```python
from build123d import *

# Parameters (mm, degrees)
CROQUIS1_W              = 52
CROQUIS1_H              = 37
SALIENTE_EXTRUIR1_DEPTH = 3
REDONDEO1_R             = 3
CROQUIS2_R              = 1.5
CORTAR_EXTRUIR1_DEPTH   = 3
CROQUIS3_W              = 29
CROQUIS3_H              = 20
CROQUIS3_W_2            = 6
CROQUIS3_H_2            = 14
CORTAR_EXTRUIR2_DEPTH   = 3
SALIENTE_EXTRUIR2_DEPTH = 9
CROQUIS5_W              = 36
CROQUIS5_H              = 28.002550662
SALIENTE_EXTRUIR3_DEPTH = 10.3
CORTAR_EXTRUIR3_START   = -28.002551
CORTAR_EXTRUIR3_DEPTH   = 28.002551
SALIENTE_EXTRUIR4_DEPTH = 8.5
CROQUIS8_W              = 21.9
CROQUIS8_H              = 60.9
CORTAR_EXTRUIR4_DEPTH   = 5.5
CORTAR_EXTRUIR5_DEPTH   = 9
CORTAR_EXTRUIR6_START   = -28.002551
CROQUIS12_W             = 9
CROQUIS12_H             = 1.570892211
CORTAR_EXTRUIR6_DEPTH   = 28.002551
CROQUIS13_W             = 3
CROQUIS13_H             = 67
SALIENTE_EXTRUIR5_DEPTH = 12
CORTAR_EXTRUIR7_START   = -28.002551
CROQUIS14_W             = 31
CROQUIS14_H             = 9
CORTAR_EXTRUIR7_DEPTH   = 28.002551
CROQUIS17_R             = 1.5
SALIENTE_EXTRUIR6_DEPTH = 9
CORTAR_EXTRUIR8_START   = -37
CROQUIS18_W             = 54.197150846
CROQUIS18_H             = 9
CORTAR_EXTRUIR8_DEPTH   = 37
CORTAR_EXTRUIR9_REACH   = 83.194
CROQUIS19_R             = 1.5
CROQUIS20_W             = 28
CROQUIS20_H             = 6
SALIENTE_EXTRUIR7_DEPTH = 3
CROQUIS21_W             = 20
CROQUIS21_H             = 4.5
CORTAR_EXTRUIR10_DEPTH  = 2
CROQUIS22_R             = 3
CORTAR_EXTRUIR11_DEPTH  = 10.3
CORTAR_EXTRUIR12_REACH  = 82.263
CROQUIS23_R             = 2


with BuildPart() as part:
    # Croquis1 → Saliente-Extruir1 (new body)
    with BuildSketch(Plane.XY):
        with Locations((-39.296803653, 6.787671233)):
            Rectangle(CROQUIS1_W, CROQUIS1_H)
    extrude(amount=SALIENTE_EXTRUIR1_DEPTH)

    # Redondeo1
    redondeo1_edges = [part.edges().sort_by_distance(p)[0] for p in [
        (-65.296803653, 25.287671233, 1.5),
        (-65.296803653, -11.712328767, 1.5),
    ]]
    fillet(redondeo1_edges, radius=REDONDEO1_R)

    # Croquis2 → Cortar-Extruir1 (cut)
    with BuildSketch(Plane.XY.offset(3)):
        with Locations((-61.296803653, 21.287671233)):
            Circle(CROQUIS2_R)
        with Locations((-61.296803653, -7.712328767)):
            Circle(CROQUIS2_R)
        with Locations((-16.624072342, -7.712328767)):
            Circle(CROQUIS2_R)
        with Locations((-17.296803653, 21.287671233)):
            Circle(CROQUIS2_R)
    extrude(amount=-CORTAR_EXTRUIR1_DEPTH, mode=Mode.SUBTRACT)

    # Croquis3 → Cortar-Extruir2 (cut)
    with BuildSketch(Plane.XY.offset(3)):
        with Locations((-50.796803653, 6.787671233)):
            Rectangle(CROQUIS3_W, CROQUIS3_H)
        with Locations((-16.296803653, 6.787671233)):
            Rectangle(CROQUIS3_W_2, CROQUIS3_H_2)
    extrude(amount=-CORTAR_EXTRUIR2_DEPTH, mode=Mode.SUBTRACT)

    # Croquis4 → Saliente-Extruir2 (add)
    with BuildSketch(Plane.XY.offset(3)):
        Polygon((-57.296803653, 16.787671233), (-57.296803653, 20.790221895), (-26.296803653, 20.790221895), (-26.296803653, -7.212328767), (-57.296803653, -7.212328767), (-57.296803653, -3.212328767), (-36.296803653, -3.212328767), (-36.296803653, 16.787671233), align=None)
    extrude(amount=SALIENTE_EXTRUIR2_DEPTH)

    # Croquis5 → Saliente-Extruir3 (add)
    with BuildSketch(Plane.XY.offset(12)):
        with Locations((-44.296803653, 6.788946564)):
            Rectangle(CROQUIS5_W, CROQUIS5_H)
    extrude(amount=SALIENTE_EXTRUIR3_DEPTH)

    # Croquis6 → Cortar-Extruir3 (cut)
    with BuildSketch(Plane.XZ.offset(7.212328767).offset(CORTAR_EXTRUIR3_START)):
        Polygon((-35.296803653, 15), (-35.296803653, 12.995381041), (-26.296803653, 12.995381041), (-26.296803653, 14.757444162), (-26.296803653, 22.3), (-62.296803653, 22.3), align=None)
    extrude(amount=CORTAR_EXTRUIR3_DEPTH, mode=Mode.SUBTRACT)

    # Croquis7 → Saliente-Extruir4 (add)
    with BuildSketch(Plane(origin=(1.374852463, 0, 5.085070754), x_dir=(0.9653390502996949, 0, -0.2609990765625102), z_dir=(0.2609990765625102, 0, 0.9653390502996949))):
        Polygon((-65.957816682, 6.788946564), (-65.957816682, -26.711053436), (-37.957816682, -26.711053436), (-37.957816682, 40.288946564), (-65.957816682, 40.288946564), align=None)
    extrude(amount=SALIENTE_EXTRUIR4_DEPTH)

    # Croquis8 → Cortar-Extruir4 (cut)
    with BuildSketch(Plane(origin=(3.593344614, 0, 13.290452681), x_dir=(0.9653390502996949, 0, -0.26099907656251026), z_dir=(0.26099907656251026, 0, 0.9653390502996949))):
        with Locations((-51.957816682, 6.788946564)):
            Rectangle(CROQUIS8_W, CROQUIS8_H)
    extrude(amount=-CORTAR_EXTRUIR4_DEPTH, mode=Mode.SUBTRACT)

    # Croquis10 → Cortar-Extruir5 (cut)
    with BuildSketch(Plane(origin=(0, 20.790221895, 0), x_dir=(1, 0, 0), z_dir=(0, 1, 0))):
        Polygon((-62.296803653, -22.3), (-35.296803653, -15), (-35.296803653, -12), (-62.296803653, -19.3), align=None)
    extrude(amount=-CORTAR_EXTRUIR5_DEPTH, mode=Mode.SUBTRACT)

    # Croquis12 → Cortar-Extruir6 (cut)
    with BuildSketch(Plane(origin=(0, 20.790221895, 0), x_dir=(1, 0, 0), z_dir=(0, 1, 0)).offset(CORTAR_EXTRUIR6_START)):
        with Locations((-30.796803653, -12.209934936)):
            Rectangle(CROQUIS12_W, CROQUIS12_H)
    extrude(amount=CORTAR_EXTRUIR6_DEPTH, mode=Mode.SUBTRACT)

    # Croquis13 → Saliente-Extruir5 (add)
    with BuildSketch(Plane(origin=(3.593344614, 0, 13.290452681), x_dir=(0.9653390502996949, 0, -0.26099907656251026), z_dir=(0.26099907656251026, 0, 0.9653390502996949))):
        with Locations((-39.457816682, 6.788946564)):
            Rectangle(CROQUIS13_W, CROQUIS13_H)
    extrude(amount=SALIENTE_EXTRUIR5_DEPTH)

    # Croquis14 → Cortar-Extruir7 (cut)
    with BuildSketch(Plane.XZ.offset(7.212328767).offset(CORTAR_EXTRUIR7_START)):
        with Locations((-41.796803653, 7.5)):
            Rectangle(CROQUIS14_W, CROQUIS14_H)
    extrude(amount=CORTAR_EXTRUIR7_DEPTH, mode=Mode.SUBTRACT)


with BuildPart() as cortar_extruir7_piece_1:
    # of the separate pieces the step leaves, piece 1, a body of its own (cortar_extruir7_pieces)
    add(part.part.solids().sort_by_distance((-62.296803653, -26.711053436, 22.3))[0])



with BuildPart() as cortar_extruir7_piece_2:
    # of the separate pieces the step leaves, piece 2, a body of its own (cortar_extruir7_pieces)
    add(part.part.solids().sort_by_distance((-62.296803653, 25.287671233, 3))[0])


with BuildPart() as cortar_extruir7_piece_1_1:
    add(cortar_extruir7_piece_1.part)

    add(cortar_extruir7_piece_2.part)  # Saliente-Extruir6 merges Cortar-Extruir7 piece 2
    # Croquis17 → Saliente-Extruir6 (add)
    with BuildSketch(Plane.XY.offset(3)):
        with BuildLine():
            Line((-13.296803653, -0.212328767), (-19.296803653, -0.212328767))
            Line((-19.296803653, -0.212328767), (-19.296803653, 13.787671233))
            Line((-19.296803653, 13.787671233), (-13.296803653, 13.787671233))
            Line((-13.296803653, 13.787671233), (-13.296803653, 25.287671233))
            Line((-13.296803653, 25.287671233), (-62.296803653, 25.287671233))
            ThreePointArc((-62.296803653, 25.287671233), (-64.418123997, 24.408991576), (-65.296803653, 22.287671233))
            Line((-65.296803653, 22.287671233), (-65.296803653, 16.787671233))
            Line((-65.296803653, 16.787671233), (-36.296803653, 16.787671233))
            Line((-36.296803653, 16.787671233), (-36.296803653, -3.212328767))
            Line((-36.296803653, -3.212328767), (-65.296803653, -3.212328767))
            Line((-65.296803653, -3.212328767), (-65.296803653, -8.712328767))
            ThreePointArc((-65.296803653, -8.712328767), (-64.418123997, -10.833649111), (-62.296803653, -11.712328767))
            Line((-62.296803653, -11.712328767), (-13.296803653, -11.712328767))
            Line((-13.296803653, -11.712328767), (-13.296803653, -0.212328767))
        make_face()
        with Locations((-61.296803653, 21.287671233)):
            Circle(CROQUIS17_R, mode=Mode.SUBTRACT)
        with Locations((-61.296803653, -7.712328767)):
            Circle(CROQUIS17_R, mode=Mode.SUBTRACT)
        with Locations((-16.624072342, -7.712328767)):
            Circle(CROQUIS17_R, mode=Mode.SUBTRACT)
        with Locations((-17.296803653, 21.287671233)):
            Circle(CROQUIS17_R, mode=Mode.SUBTRACT)
    extrude(amount=SALIENTE_EXTRUIR6_DEPTH)

    # Croquis18 → Cortar-Extruir8 (cut)
    with BuildSketch(Plane.XZ.offset(11.712328767).offset(CORTAR_EXTRUIR8_START)):
        with Locations((-40.395379076, 4.5)):
            Rectangle(CROQUIS18_W, CROQUIS18_H)
    extrude(amount=CORTAR_EXTRUIR8_DEPTH, mode=Mode.SUBTRACT)

    # Cortar-Extruir9: up to this plane
    cortar_extruir9_end = Plane(origin=(3.593344614, 0, 13.290452681), z_dir=(0.26099907656251026, 0, 0.9653390502996949))
    # Croquis19 → Cortar-Extruir9 (cut, up to the surface)
    with BuildSketch(Plane(origin=(0, 0, 9), x_dir=(-1, 0, 0), z_dir=(0, 0, -1)), mode=Mode.PRIVATE) as cortar_extruir9_sk1:
        with Locations(Location((61.296803653, 21.287671233, 0), (0, 0, 180))):
            Circle(CROQUIS19_R)
    cortar_extruir9_tool1 = split(extrude(cortar_extruir9_sk1.sketch, amount=-CORTAR_EXTRUIR9_REACH, mode=Mode.PRIVATE), bisect_by=cortar_extruir9_end, keep=Keep.BOTH, mode=Mode.PRIVATE)
    add(cortar_extruir9_tool1.solids().sort_by_distance((-61.296804, 21.287671, 9))[0], mode=Mode.SUBTRACT)
    # Croquis19 → Cortar-Extruir9 (cut, up to the surface)
    with BuildSketch(Plane(origin=(0, 0, 9), x_dir=(-1, 0, 0), z_dir=(0, 0, -1)), mode=Mode.PRIVATE) as cortar_extruir9_sk2:
        with Locations(Location((61.296803653, -7.712328767, 0), (0, 0, 180))):
            Circle(CROQUIS19_R)
    cortar_extruir9_tool2 = split(extrude(cortar_extruir9_sk2.sketch, amount=-CORTAR_EXTRUIR9_REACH, mode=Mode.PRIVATE), bisect_by=cortar_extruir9_end, keep=Keep.BOTH, mode=Mode.PRIVATE)
    add(cortar_extruir9_tool2.solids().sort_by_distance((-61.296804, -7.712329, 9))[0], mode=Mode.SUBTRACT)

    # Croquis20 → Saliente-Extruir7 (add)
    with BuildSketch(Plane(origin=(1.374852463, 0, 5.085070754), x_dir=(-0.9653390502996949, 0, 0.26099907656251026), z_dir=(-0.26099907656251026, 0, -0.9653390502996949))):
        with Locations((51.957816682, 37.288946564)):
            Rectangle(CROQUIS20_W, CROQUIS20_H)
    extrude(amount=SALIENTE_EXTRUIR7_DEPTH)

    # Croquis21 → Cortar-Extruir10 (cut)
    with BuildSketch(Plane(origin=(0, 0, 9), x_dir=(-1, 0, 0), z_dir=(0, 0, -1))):
        with Locations((45.296803653, 19.037671233)):
            Rectangle(CROQUIS21_W, CROQUIS21_H)
        with Locations((45.296803653, -5.462328767)):
            Rectangle(CROQUIS21_W, CROQUIS21_H)
    extrude(amount=-CORTAR_EXTRUIR10_DEPTH, mode=Mode.SUBTRACT)

    # Croquis22 → Cortar-Extruir11 (cut)
    with BuildSketch(Plane.XY.offset(12)):
        with Locations((-61.296803653, 21.287671233)):
            Circle(CROQUIS22_R)
        with Locations((-61.296803653, -7.712328767)):
            Circle(CROQUIS22_R)
    extrude(amount=CORTAR_EXTRUIR11_DEPTH, mode=Mode.SUBTRACT)

    # Cortar-Extruir12: up to this plane
    cortar_extruir12_end = Plane(origin=(3.593344614, 0, 13.290452681), z_dir=(0.26099907656251026, 0, 0.9653390502996949))
    # Croquis23 → Cortar-Extruir12 (cut, up to the surface)
    with BuildSketch(Plane.XY.offset(12), mode=Mode.PRIVATE) as cortar_extruir12_sk1:
        with Locations((-61.296803653, 21.287671233)):
            Circle(CROQUIS23_R)
    cortar_extruir12_tool1 = split(extrude(cortar_extruir12_sk1.sketch, amount=CORTAR_EXTRUIR12_REACH, mode=Mode.PRIVATE), bisect_by=cortar_extruir12_end, keep=Keep.BOTH, mode=Mode.PRIVATE)
    add(cortar_extruir12_tool1.solids().sort_by_distance((-61.296804, 21.287671, 12))[0], mode=Mode.SUBTRACT)
    # Croquis23 → Cortar-Extruir12 (cut, up to the surface)
    with BuildSketch(Plane.XY.offset(12), mode=Mode.PRIVATE) as cortar_extruir12_sk2:
        with Locations((-61.296803653, -7.712328767)):
            Circle(CROQUIS23_R)
    cortar_extruir12_tool2 = split(extrude(cortar_extruir12_sk2.sketch, amount=CORTAR_EXTRUIR12_REACH, mode=Mode.PRIVATE), bisect_by=cortar_extruir12_end, keep=Keep.BOTH, mode=Mode.PRIVATE)
    add(cortar_extruir12_tool2.solids().sort_by_distance((-61.296804, -7.712329, 12))[0], mode=Mode.SUBTRACT)


solid = cortar_extruir7_piece_1_1.part
```
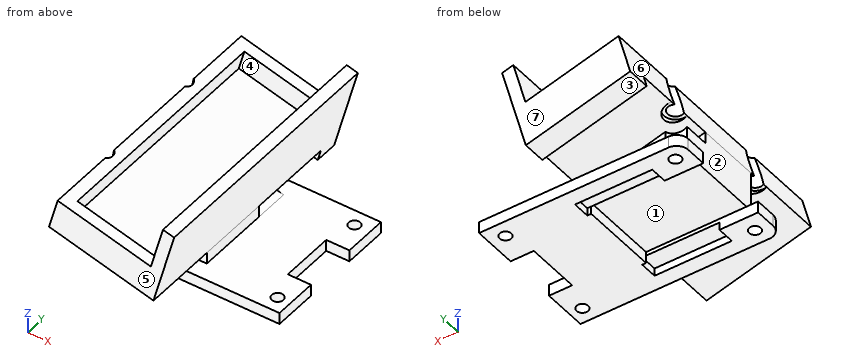
Can you work these out from the model? Positions are in its coordinate system, mm. Face numbers are marked on the shaded views. A direction names the side the tool comes from. Round coordinates to 2 decimals unless told otherwise and drop trailing zeros. Loops run counter-clockwise (first coordinate to the right, second up) from the corner with the lowest first, then second, coordinate; pieces in that order, holes last. Notation, with made-up numbers: M 85,46.5 L 115,46.5 A23 ccw 115,73.5 Z; hole C 0.5,59.25 d6. An arc over 180 degrees is marked long. Answer as a JSON object with one key per item and string values. Group by question number.
Q1. On a 3-axis mill with a long thin cutter (end or side, diameter ignored), from which of +Z, -Z, +X, -X, +Y, -Y can I reach the whole of each face in a straight line? I mean the marked faces 1, 2 and 3. Say none if no direction works.
Q2. Imagine slicing it at A-A, the plane y = 16. Please give me the cut outline in (x, z).
Q3. Imagine slicing it at D-D, the plane x = -52. Please give me the cut outline in (y, z).
Q4. We'd pull the mould along Y, two halves only. Please class the marked faces 4, 5, 6 and 7: +Y half, -Y half, draft (parallel to the pull), parting line (faces both ways), or undercut.
Q5. Imagine slicing it at C-C, the plane x = -40. Please give me the cut outline in (y, z), then the cut area to 3 significant figures.
Q6. Imagine slicing it at B-B, the plane y = 35. Please give me the cut outline in (x, z).
Q7. Please list where these lines run through material, in increasing order: L1, parallel to Y at x = -55, z = 28.5; L2, parallel to Y at x = -50.5, z = 12.5; L3, parallel to X at y = -16.5, z = 28.
Q8. Will these pins go through, and if not, where does the flat tip stop? pin 1 (6 mm diameter, centred on x = -55, y = 3.5, fed in from -Z); pin 2 (3 mm diameter, centred on x = -46.5, z = 14.5, fed in from +Y); pin 3 (1.5 mm diameter, centred on x = -41.5, z = 13.5, fed in from -Y); pin 4 (12 mm diameter, centred on x = -22.5, y = -13.5, fed in from +Z).
Findings:
{
 "1": {"face 1": "-Z, -X", "face 2": "+Z, -X, -Y", "face 3": "-Z, -X, +Y"},
 "2": {"outline": "M -62.3,12 L -36.3,12 L -36.3,9 L -13.3,9 L -13.3,12 L -35.3,12 L -62.3,19.3 Z; M -62.3,22.3 L -35.27,14.99 L -29.92,34.78 L -32.81,35.56 L -35.94,23.98 L -35.99,23.99 L -37.43,18.68 L -58.57,24.4 L -57.13,29.71 L -60.08,30.51 Z"},
 "3": {"outline": "M -26.71,19.52 L -7.21,19.52 L -7.21,12 L -11.71,12 L -11.71,9 L -7.71,9 L -7.71,11 L -3.21,11 L -3.21,12 L 16.79,12 L 16.79,11 L 21.29,11 L 21.29,9 L 25.29,9 L 25.29,12 L 20.79,12 L 20.79,16.52 L 11.79,16.52 L 11.79,19.52 L 34.29,19.52 L 34.29,16.41 L 40.29,16.41 L 40.29,28.32 L 37.24,28.32 L 37.24,22.62 L -23.66,22.62 L -23.66,28.32 L -26.71,28.32 Z"},
 "4": {"face 4": "undercut", "face 5": "-Y half", "face 6": "draft", "face 7": "+Y half"},
 "5": {"outline": "M -26.71,16.27 L -7.21,16.27 L -7.21,12 L -11.71,12 L -11.71,9 L -7.71,9 L -7.71,11 L -3.21,11 L -3.21,12 L 16.79,12 L 16.79,11 L 21.29,11 L 21.29,9 L 25.29,9 L 25.29,12 L 20.79,12 L 20.79,13.27 L 11.79,13.27 L 11.79,16.27 L 34.29,16.27 L 34.29,13.16 L 40.29,13.16 L 40.29,25.08 L 37.24,25.08 L 37.24,19.38 L -23.66,19.38 L -23.66,25.08 L -26.71,25.08 Z", "area": "387 mm2"},
 "6": {"outline": "M -63.08,19.4 L -36.05,12.1 L -29.92,34.78 L -32.81,35.56 L -35.94,23.98 L -35.99,23.99 L -37.43,18.68 L -58.57,24.4 L -57.13,29.71 L -60.08,30.51 Z"},
 "7": {"L1": "y = -26.71 to -23.66, 37.24 to 40.29", "L2": "y = -7.21 to 20.79", "L3": "x = -60.76 to -57.6, -34.86 to -31.75"},
 "8": {"pin 1": "stops at z = 12", "pin 2": "stops at y = 40.29", "pin 3": "stops at y = -7.21", "pin 4": "stops at z = 12"}
}
